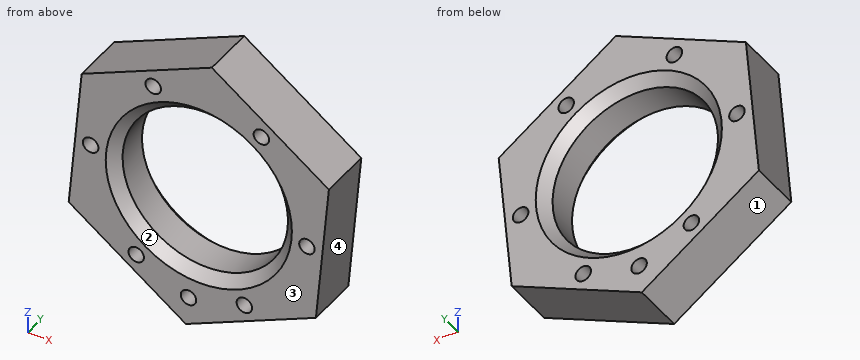
```python
from build123d import *

# Parameters (mm, degrees)
BOSS_EXTRUDE1_DEPTH = 6.35
SKETCH2_R           = 10.16
CUT_EXTRUDE1_DEPTH  = 25.548672232
CHAMFER1_SIZE       = 1.27
SKETCH4_R           = 0.9525
CUT_EXTRUDE2_DEPTH  = 25.548672232


with BuildPart() as part:
    # Sketch1 → Boss-Extrude1 (new body)
    with BuildSketch(Plane(origin=(0, 0, 0), x_dir=(1, 0, 0), z_dir=(0, 1, 0))):
        Polygon((1.59389926, -17.525304139), (15.974308223, -7.382294819), (14.380408963, 10.143009319), (-1.59389926, 17.525304139), (-15.974308223, 7.382294819), (-14.380408963, -10.143009319), align=None)
    extrude(amount=BOSS_EXTRUDE1_DEPTH)

    # Sketch2 → Cut-Extrude1 (cut, through all)
    with BuildSketch(Plane(origin=(0, 6.35, 0), x_dir=(1, 0, 0), z_dir=(0, 1, 0))):
        with Locations(Location((0, 0, 0), (0, 0, 270))):
            Circle(SKETCH2_R)
    extrude(amount=-CUT_EXTRUDE1_DEPTH, mode=Mode.SUBTRACT)

    # Chamfer1
    chamfer1_edges = [part.edges().sort_by_distance(p)[0] for p in [
        (0, 0, -10.16),
        (0, 6.35, -10.16),
    ]]
    chamfer(chamfer1_edges, length=CHAMFER1_SIZE)

    # Sketch4 → Cut-Extrude2 (cut, through all)
    with BuildSketch(Plane(origin=(0, 6.35, 0), x_dir=(1, 0, 0), z_dir=(0, 1, 0))):
        with Locations(Location((-7.686090774, 10.897074544, 0), (0, 0, 270))):
            Circle(SKETCH4_R)
        with Locations(Location((5.594097995, 12.104887138, 0), (0, 0, 270))):
            Circle(SKETCH4_R)
        with Locations(Location((13.280188769, 1.207812594, 0), (0, 0, 270))):
            Circle(SKETCH4_R)
        with Locations(Location((7.686090774, -10.897074544, 0), (0, 0, 270))):
            Circle(SKETCH4_R)
        with Locations(Location((-5.594097995, -12.104887138, 0), (0, 0, 270))):
            Circle(SKETCH4_R)
        with Locations(Location((-1.265327479, 13.91257871, 0), (0, 0, 270))):
            Circle(SKETCH4_R)
        with Locations(Location((-13.280188769, -1.207812594, 0), (0, 0, 270))):
            Circle(SKETCH4_R)
    extrude(amount=-CUT_EXTRUDE2_DEPTH, mode=Mode.SUBTRACT)


solid = part.part
```
Geometry check sheet. Reference: the model listing, model coordinates, mm. Face numbers are marked on the shaded views. Coordinates: 2 decimals unless noted, no trailing zeros. Write each loop counter-clockwise with the first axis right and the second up, starting at its lowest first coordinate (ties: lowest second). Pieces come first, ordered by that corner, then holes. Notation, with made-up numbers: M 76,48 L 108,48 A20 cw 108,71 Z; hole C 61.25,52.5 d10. An arc over 180 degrees is marked long. One line per item, written item: value. Start each with the question number.
(1) Release check for a two-part mould opening along X. For the marked faces 1, 2, 3 and 4 record: released by +X, released by -X, zero draft, split by the parting line, or undercut.
(2) Sectioned sample at B-B, the plane y = 2. State how many separate pieces and enclosed holes the cut face has, and give its area (3 significant figures).
(3) Scan lines: line 1 along Z through (x, y) = (-5.5, 2.5); line 2 along Z through (x, y) = (-8.5, 1.5); line 3 along X through (y, z) = (6.25, -9). Record each from-to range of solid material in increasing order. Write a range as [from, to].
(4) Depth check by flat-ended pin: pin 1 (1.5 mm diameter, centred on x = -3.5, y = 4.5, fed in from +Z); pin 2 (1.1 mm diameter, centred on x = 5.59, z = -12.1, fed in from +Y); pin 3 (1.5 mm diameter, centred on x = 4.5, y = 3.5, fed in from -Z); pin 4 (1 mm diameter, centred on x = -6, y = 3.5, fed in from -Z). Enter the tip coordinate at first touch or a pass-through.
(5) Sectioned sample at A-A, the plane z = -14. Enter the section's corners in (x, y), and give its area (3 significant figures).
Filled sheet:
1. face 1: released by -X
1. face 2: undercut
1. face 3: zero draft
1. face 4: released by +X
2. separate pieces: 1
2. enclosed holes: 8
2. area: 460 mm²
3. line 1: [-14.77, -8.54], [8.54, 11.16], [13.05, 14.25]
3. line 2: [-12.65, -11.39], [-10.4, -5.57], [5.57, 12.86]
3. line 3: [-13.68, -6.88], [6.88, 14.48]
4. pin 1: z = 15.52
4. pin 2: through
4. pin 3: z = -15.06
4. pin 4: z = -14.77
5. outline: M -6.59,0 L -2.21,0 L -2.21,6.35 L -6.59,6.35 Z; M -0.32,0 L 6.03,0 L 6.03,6.35 L -0.32,6.35 Z
5. area: 68.1 mm²
